Design review of the part built by this model. Coordinates are the model's own, in mm. A direction names the side the tool comes from. Give positions to 0.01 mm unless a question says otherwise; leave off trailing zeros. Write each loop counter-clockwise with the first axis right and the second up, starting at its lowest first coordinate (ties: lowest second). Pieces come first, ordered by that corner, then holes.
```python
from build123d import *

# Parameters (mm, degrees)
BOSS_EXTRU_1_DEPTH           = 104
ENL_V_MAT_EXTRU_1_DEPTH      = 143.789209242
ENL_V_MAT_EXTRU_1_DEPTH_BACK = 143.789209242
ESQUISSE4_R                  = 25
ENL_V_MAT_EXTRU_2_DEPTH      = 173.617375359
CONG_1_R                     = 15


with BuildPart() as part:
    # Esquisse1 → Boss.-Extru.1 (new body)
    with BuildSketch(Plane.XY):
        Polygon((80.229410292, 56), (-23.770589708, 56), (0, 0), (56.458820585, 0), align=None)
        Polygon((-23.770589708, -56), (0, 0), (56.458820585, 0), (80.229410292, -56), align=None)
    extrude(amount=BOSS_EXTRU_1_DEPTH)

    # Esquisse3 → Enlèv. mat.-Extru.1 (cut, two sides: drawn at the far end of the back side and taken through both)
    with BuildSketch(Plane(origin=(0, 0, 0), x_dir=(0, 0, -1), z_dir=(1, 0, 0)).offset(-ENL_V_MAT_EXTRU_1_DEPTH_BACK)):
        Polygon((-23.770589708, 0), (0, 0), (0, 56), align=None)
        Polygon((0, 0), (0, -56), (-23.770589708, 0), align=None)
        Polygon((-104, 0), (-104, 56), (-80.229410292, 0), align=None)
        Polygon((-80.229410292, 0), (-104, 0), (-104, -56), align=None)
    extrude(amount=ENL_V_MAT_EXTRU_1_DEPTH + ENL_V_MAT_EXTRU_1_DEPTH_BACK, mode=Mode.SUBTRACT)

    # Esquisse4 → Enlèv. mat.-Extru.2 (cut, through all)
    with BuildSketch(Plane(origin=(0, 56, 0), x_dir=(1, 0, 0), z_dir=(0, 1, 0))):
        with Locations(Location((31.437518052, -50, 0), (0, 0, 180))):
            Circle(ESQUISSE4_R)
    extrude(amount=-ENL_V_MAT_EXTRU_2_DEPTH, mode=Mode.SUBTRACT)

    # Congé1
    cong_1_edges = [part.edges().sort_by_distance(p)[0] for p in [
        (56.458820585, 0, 52),
        (0, 0, 52),
        (28.229410292, 0, 23.770589708),
        (28.229410292, 0, 80.229410292),
    ]]
    fillet(cong_1_edges, radius=CONG_1_R)


solid = part.part
```
(1) To check wall thickness, follow L1, parallel to Z at x = 43, y = 46.5; L2, parallel to Y at x = 73, z = 15; L3, parallel to Y at x = 75.5, z = 73. State the ranges of each line that lie inside material, in increasing order.
Resolved:
L1: z = 4.03 to 27.83, 72.17 to 99.97
L2: y = -56 to -38.97, 38.97 to 56
L3: y = -56 to -44.86, 44.86 to 56
(2) Consider section A-A, the plane z = 50. Give the boundary of the cut face in (x, y).
Resolved:
outline: (-23.77, -56) - (6.44, -56) - (6.44, 56) - (-23.77, 56) - (-2.49, 5.86) arc R15 cw to (-2.49, -5.86) - close; (56.44, -56) - (80.23, -56) - (58.95, -5.86) arc R15 cw to (58.95, 5.86) - (80.23, 56) - (56.44, 56) - close
(3) Consider section D-D, the plane z = 16.5. Give the boundary of the cut face in (x, y).
Resolved:
outline: (-23.77, -56) - (80.23, -56) - (63.73, -17.13) - (-7.27, -17.13) - close; (-23.77, 56) - (-7.27, 17.13) - (63.73, 17.13) - (80.23, 56) - close
(4) Mouldability with a two-part tool opening along X and no side actions: class faces 4 (the face through (51.28, 0.78, 34.79)), 5 (the face through (6, -56, 51)), 6 (the face through (-13.278, -31.281, 51.272)) as pulls with the +X half, pulls with the -X half, needs draft (parallel to the pull), parting line crosses it, or undercut.
Resolved:
face 4: undercut
face 5: needs draft
face 6: pulls with the -X half
(5) Consider section C-C, the plane y = -34. Give the boundary of the cut face in (x, z), then the cut area to 3 significant figures.
Resolved:
outline: (-14.43, 9.34) - (70.89, 9.34) - (70.89, 94.66) - (-14.43, 94.66) - close; hole circle Ø50 at (31.44, 50)
area: 5,320 mm2
(6) Tool access review of faces 1 (the face through (27.501, 31.281, 10.492)), 2 (the face through (27.501, -31.281, 93.508)), 3 (the face through (69.44, -30.58, 51.27)): name each direction out of +Z, -Z, +X, -X, +Y, -Y from which nothing blocks a thin tool from reaching the whole face with its end or side.
Resolved:
face 1: -Z, +X, -X
face 2: +Z, +X, -X
face 3: +Z, -Z, +X
(7) Consider section B-B, the plane x = 32. Give the boundary of the cut face in (y, z), then the cut area to 3 significant figures.
Resolved:
outline: (-56, 0) - (-5.86, 21.28) arc R15 cw to (5.86, 21.28) - (56, 0) - (56, 25.01) - (-56, 25.01) - close; (-56, 74.99) - (56, 74.99) - (56, 104) - (5.86, 82.72) arc R15 cw to (-5.86, 82.72) - (-56, 104) - close
area: 3,400 mm2
(8) Clearance check with flat-ended pins moving along their axes: P1, Ø1.5, axis at x = -5, y = 5, coming from the -Z side; P2, Ø1.5, axis at x = 14.5, y = -30.5, coming from the -Z side; P3, Ø1.5, axis at x = 30.5, y = -5.5, coming from the +Z side; P4, Ø1.5, axis at y = -44.5, z = 80.5, coming from the -X side. State where each tip first meets the part, or that it passes through.
Resolved:
P1: passes through
P2: stops at z = 10.51
P3: stops at z = 82.88
P4: stops at x = -19.21
